```python
from build123d import *

# Parameters (mm, degrees)
F0_R     = 1.5
F0_R_2   = 11.025
F1_DEPTH = 5.5
F0_R_3   = 9
F2_DEPTH = 2
F3_R     = 2


with BuildPart() as f1:
    # F0 (on Top) → F1 (new body)
    with BuildSketch(Plane.XY):
        with BuildLine():
            ThreePointArc((-12.1141484076, -3.0817865531), (-15.3023705753, -8.8348277709), (-8.7259796478, -8.9502669896))
            ThreePointArc((-8.7259796478, -8.9502669896), (-10.8253175473, -6.25), (-12.1141484076, -3.0817865531))
        make_face()
        with Locations((-12.7438917843, -7.3576893522)):
            Circle(F0_R, mode=Mode.SUBTRACT)
        with BuildLine():
            ThreePointArc((12.1141484076, -3.0817865531), (12.403161998, -1.5529238399), (12.5, 0))
            ThreePointArc((12.5, 0), (9.9649914575, 7.5464524945), (3.3881687598, 12.0320535427))
            ThreePointArc((3.3881687598, 12.0320535427), (1.7101653013, 12.3824607668), (0, 12.5))
            ThreePointArc((0, 12.5), (-1.7101653013, 12.3824607668), (-3.3881687598, 12.0320535427))
            ThreePointArc((-3.3881687598, 12.0320535427), (-10.8253175473, 6.25), (-12.1141484076, -3.0817865531))
            ThreePointArc((-12.1141484076, -3.0817865531), (-10.8253175473, -6.25), (-8.7259796478, -8.9502669896))
            ThreePointArc((-8.7259796478, -8.9502669896), (0, -12.5), (8.7259796478, -8.9502669896))
            ThreePointArc((8.7259796478, -8.9502669896), (10.8253175473, -6.25), (12.1141484076, -3.0817865531))
        make_face()
        Circle(F0_R_2, mode=Mode.SUBTRACT)
        with BuildLine():
            ThreePointArc((-3.3881687598, 12.0320535427), (-1.7101653013, 12.3824607668), (0, 12.5))
            Line((0, 12.5), (0, 13.2153787043))
            ThreePointArc((0, 13.2153787043), (-1.5, 14.7153787043), (0, 16.2153787043))
            Line((0, 16.2153787043), (0, 16.9307574087))
            Line((0, 16.9307574087), (0, 17.6696555418))
            ThreePointArc((0, 17.6696555418), (-3.2887020177, 15.8092112452), (-3.3881687598, 12.0320535427))
        make_face()
        with BuildLine():
            ThreePointArc((0, 12.5), (1.7101653013, 12.3824607668), (3.3881687598, 12.0320535427))
            ThreePointArc((3.3881687598, 12.0320535427), (3.2887020177, 15.8092112452), (0, 17.6696555418))
            Line((0, 17.6696555418), (0, 16.9307574087))
            Line((0, 16.9307574087), (0, 16.2153787043))
            ThreePointArc((0, 16.2153787043), (1.0606601718, 15.7760388761), (1.5, 14.7153787043))
            ThreePointArc((1.5, 14.7153787043), (1.0606601718, 13.6547185326), (0, 13.2153787043))
            Line((0, 13.2153787043), (0, 12.5))
        make_face()
        with BuildLine():
            ThreePointArc((8.7259796478, -8.9502669896), (15.3023705753, -8.8348277709), (12.1141484076, -3.0817865531))
            ThreePointArc((12.1141484076, -3.0817865531), (10.8253175473, -6.25), (8.7259796478, -8.9502669896))
        make_face()
        with Locations((12.7438917843, -7.3576893522)):
            Circle(F0_R, mode=Mode.SUBTRACT)
    extrude(amount=F1_DEPTH)

    # F0 (on Top) → F2 (join)
    with BuildSketch(Plane.XY):
        Circle(F0_R_2)
        Circle(F0_R_3, mode=Mode.SUBTRACT)
    extrude(amount=F2_DEPTH)

    # F3
    f3_edges = [f1.edges().sort_by_distance(p)[0] for p in [
        (3.388169, 12.032054, 2.75),
        (8.72598, -8.950267, 2.75),
        (-12.114148, -3.081787, 2.75),
        (-8.72598, -8.950267, 2.75),
        (-3.388169, 12.032054, 2.75),
        (12.114148, -3.081787, 2.75),
    ]]
    fillet(f3_edges, radius=F3_R)


solid = f1.part
```
CAD build for the part. Positions are in the model's coordinates, mm. A direction names the side the tool comes from. Coordinates: 2 decimals unless noted, no trailing zeros. Order: outer loops, then holes, each group sorted by start corner. A loop starts at its lowest first (then second) coordinate and runs counter-clockwise, first axis right, second up. Notation, with made-up numbers: (-8.5, 11.5) -> (5.5, 11.5) arc R36 ccw to (5.5, 47.5) -> close; hole circle Ø5 at (17, 17.25). An arc over 180 degrees is marked (long way). Use one line per item in the form item = value. Start each with the question number.
1) Drop flat-ended pins along their axis: pin 1 (3 mm diameter, centred on x = 6, z = 4.5, fed in from +Y); pin 2 (1.5 mm diameter, centred on y = 5.5, z = 4, fed in from +X); pin 3 (1 mm diameter, centred on y = 1.5, z = 2.5, fed in from -X). Give the stop position or say it passes through.
2) Band-saw the part on C-C on x = 3. Give the cut face in (y, z).
3) Drill centre lines: L1, parallel to X at y = -6.5, z = 0.55; L2, parallel to Y at x = 0.5, z = 1.95; L3, parallel to X at y = 8, z = 0.6. Where is each one in solid material? Low to high. Write a range as [from, to].
4) Band-saw the part on A-A on x = -12. Give the cut face in (y, z).
5) Band-saw the part on B-B on z = 0.8. State how many separate pieces and enclosed holes the cut face has, then the cut area to 3 significant figures.
6) Pull direction X, two halves, no side cores. Call faces 1 (the cylindrical face through (-2.39, -10.763, 3.726)), 2 (the flat face through (-6, -10, 5.5)), 3 (the cylindrical face through (-10.769, 6.346, 2.712)), 4 (the cylindrical face through (-0.1, -12.5, 2.7)): +X half, -X half, draft (parallel to the pull), parting line (faces both ways), or undercut.
7) Tool access for faces 5 (the cylindrical face through (-11.94, -6.09, 2.71)), 6 (the flat face through (2, -9, 2)): list every direction of +Z, -Z, +X, -X, +Y, -Y with a clear straight run to the whole face (end or side of a thin tool).
Entries:
q1.pin_1 = 11.77
q1.pin_2 = 11.56
q1.pin_3 = -12.46
q2.outline = (-12.13, 0) -> (-8.49, 0) -> (-8.49, 2) -> (-10.61, 2) -> (-10.61, 5.5) -> (-12.13, 5.5) -> close; (8.49, 0) -> (16.22, 0) -> (16.22, 5.5) -> (10.61, 5.5) -> (10.61, 2) -> (8.49, 2) -> close
q3.L1 = [-15.79, -13.97], [-11.51, -6.22], [6.22, 11.51], [13.97, 15.79]
q3.L2 = [-12.49, -8.99], [8.99, 13.3], [16.13, 17.64]
q3.L3 = [-9.6, -4.12], [4.12, 9.6]
q4.outline = (-10.75, 0) -> (-8.66, 0) -> (-8.66, 5.5) -> (-10.75, 5.5) -> close; (-6.06, 0) -> (3.5, 0) -> (3.5, 5.5) -> (-6.06, 5.5) -> close
q5.separate_pieces = 1
q5.enclosed_holes = 4
q5.area = 322 mm2
q6.face_1 = undercut
q6.face_2 = draft
q6.face_3 = -X half
q6.face_4 = undercut
q7.face_5 = +Z, -Z
q7.face_6 = +Z
